```python
from build123d import *

# Parameters (mm, degrees)
F2_R     = 10.323596
F3_DEPTH = 36.068
F4_SIZE  = 5.08


with BuildPart() as f1:
    # F0 (on Front) → F1 (revolve)
    with BuildSketch(Plane.XZ):
        Polygon((0, 208.260372), (0, 0), (28.794192, 0), (28.794192, 135.701105), (14.397096, 135.701105), (14.397096, 149.391532), (28.794192, 149.391532), (28.794192, 163.081944), (14.397096, 163.081944), (14.397096, 176.772371), (28.794192, 176.772371), (28.794192, 191.831857), (14.397096, 191.831857), (28.794192, 208.260372), align=None)
        Polygon((28.794192, 0), (0, 0), (0, -208.260372), (28.794192, -208.260372), (14.397096, -191.831857), (28.794192, -191.831857), (28.794192, -176.772371), (14.397096, -176.772371), (14.397096, -163.081944), (28.794192, -163.081944), (28.794192, -149.391532), (14.397096, -149.391532), (14.397096, -135.701105), (28.794192, -135.701105), align=None)
    revolve(axis=Axis((0, 0, -104.130186), (0, 0, -1)))

    # F2 (on Front) → F3 (join)
    with BuildSketch(Plane.XZ):
        with Locations((0, 93.211494)):
            Circle(F2_R)
        with Locations((0, -93.211494)):
            Circle(F2_R)
    extrude(amount=F3_DEPTH)

    # F4
    f4_edges = [f1.edges().sort_by_distance(p)[0] for p in [
        (-10.323596, -36.068, 93.211494),
        (-10.323596, -36.068, -93.211494),
    ]]
    chamfer(f4_edges, length=F4_SIZE)


solid = f1.part
```
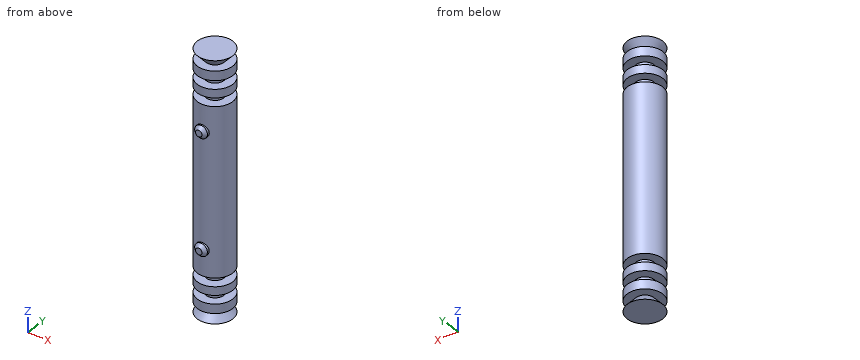
Geometry: final body of the model. Coordinates: model frame, mm. Round coordinates to 2 decimals unless told otherwise and drop trailing zeros. Order: outer loops, then holes, each group sorted by start corner. A loop starts at its lowest first (then second) coordinate and runs counter-clockwise, first axis right, second up. Notation, with made-up numbers: (72.25, 45.25) -> (129.25, 45.25) arc R20 ccw to (129.25, 70.25) -> close; hole circle Ø6 at (76, 2). An arc over 180 degrees is marked (long way). Use one line per item in the form item = value. Start each with the question number.
1. Cut plane B-B (z = 9). Return the cut outline in (x, y).
2. Pin query (flat end, axial travel): pin 1 Ø4 at (x, z) = (1, 1) entering from +Y; pin 2 Ø4 at (x, z) = (0, 72) entering from -Y; pin 3 Ø1.5 at (y, z) = (-2, -111) entering from +X; pin 4 Ø1 at (y, z) = (18.5, -137) entering from +X. Return the tip coordinate at first contact, or that it passes through.
3. Cut plane A-A (y = 18.5). Count the separate pieces of the cut face and the enclosed holes in it, then the cut area to 3 significant figures.
4. Line query: probe 1 along Y at (x, z) = (-2, -108); probe 2 along X at (y, z) = (6, 7); probe 3 along Y at (x, z) = (4.5, 100.5). Output: solid intervals per line, ascending.
Solution:
q1.outline = circle Ø57.59 at (0, 0)
q2.pin_1 = 28.79
q2.pin_2 = -28.79
q2.pin_3 = 28.77
q2.pin_4 = through
q3.separate_pieces = 7
q3.enclosed_holes = 0
q3.area = 15,200 mm^2
q4.probe_1 = -28.72 to 28.72
q4.probe_2 = -28.16 to 28.16
q4.probe_3 = -32.75 to 28.44
